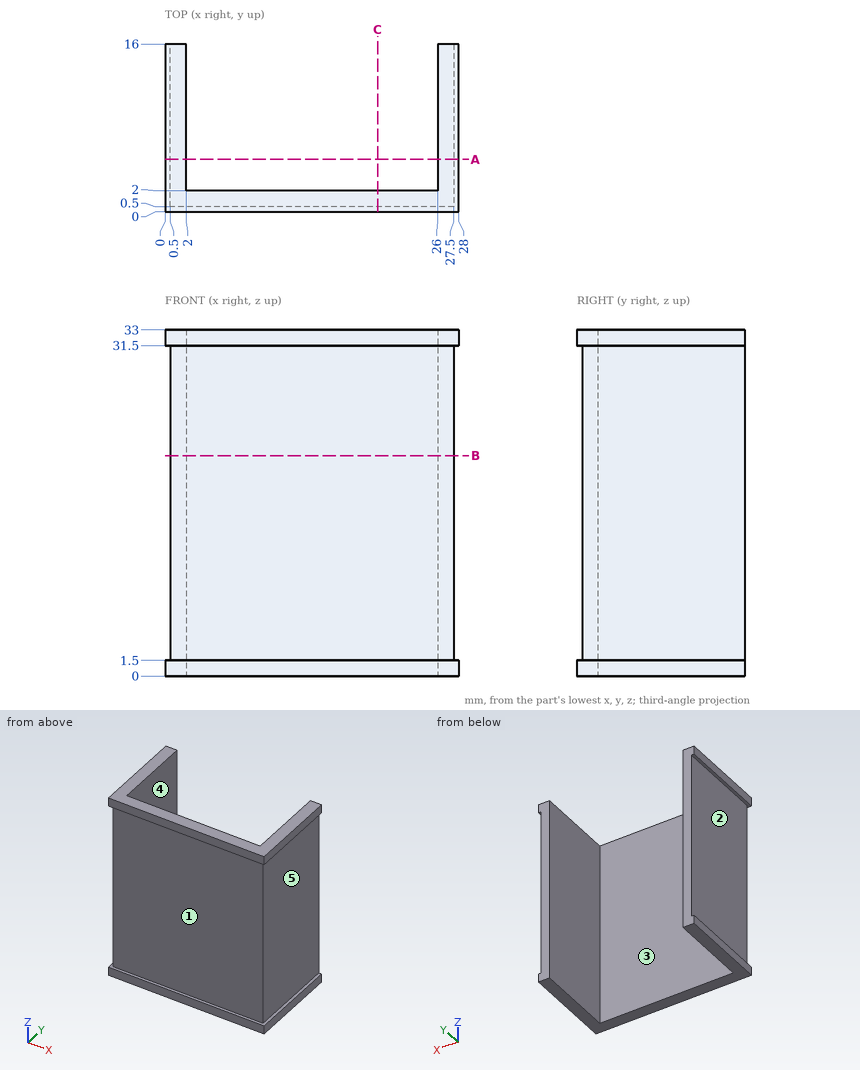
For this review, use the dimensioned drawing (mm, ordinates from the lowest corner) and the shaded views. A direction names the side the tool comes from. Coordinates: 2 decimals unless noted, no trailing zeros. Loops run counter-clockwise (first coordinate to the right, second up) from the corner with the lowest first, then second, coordinate; pieces in that order, holes last.
1. Insertion check: P1, Ø5, axis at y = 3.5, z = 11.5, coming from the -X side; P2, Ø8, axis at x = 11, z = 4.5, coming from the +Y side; P3, Ø1.5, axis at x = 8.5, z = 8, coming from the -Y side. Each pin has a flat end and moves straight along its axis. Give the tip position at first contact, or say it passes through.
2. Add section B-B, the plane z = 21. Give the boundary of the cut face in (x, y), then the cut area to 3 significant figures.
3. For the marked faces 4 and 5, list the 3-axis set-ups (+Z, -Z, +X, -X, +Y, -Y) from which the entire face can be reached by the end or side of a thin tool; tool diameter is ignored.
4. For line 1 (X direction, y = 9.5, z = 6); line 2 (Y direction, x = 23.5, z = 4); line 3 (Y direction, x = 26.5, z = 11), list the stretches that pass through material, from the lowest coordinate up.
5. Add section C-C, the plane x = 20.25. Give the boundary of the cut face in (y, z), then the cut area to 3 significant figures.
6. Mouldability with a two-part tool opening along Z and no side actions: class the marked faces 1, 2 and 3 as +Z half, -Z half, draft (parallel to the pull), parting line (faces both ways), or undercut.
7. Add section A-A, the plane y = 5. Give the boundary of the cut face in (x, z), then the cut area to 3 significant figures.
Result:
1. P1: stops at x = 0.5
1. P2: stops at y = 2
1. P3: stops at y = 0.5
2. outline: (0.5, 0.5) - (27.5, 0.5) - (27.5, 16) - (26, 16) - (26, 2) - (2, 2) - (2, 16) - (0.5, 16) - close
2. area: 82.5 mm2
3. face 4: +Z, -Z, +Y
3. face 5: +X, +Y, -Y
4. line 1: x = 0.5 to 2, 26 to 27.5
4. line 2: y = 0.5 to 2
4. line 3: y = 0.5 to 16
5. outline: (0, 0) - (2, 0) - (2, 33) - (0, 33) - (0, 31.5) - (0.5, 31.5) - (0.5, 1.5) - (0, 1.5) - close
5. area: 51.0 mm2
6. face 1: undercut
6. face 2: undercut
6. face 3: draft
7. outline: (0, 0) - (2, 0) - (2, 33) - (0, 33) - (0, 31.5) - (0.5, 31.5) - (0.5, 1.5) - (0, 1.5) - close; (26, 0) - (28, 0) - (28, 1.5) - (27.5, 1.5) - (27.5, 31.5) - (28, 31.5) - (28, 33) - (26, 33) - close
7. area: 102 mm2
